```python
from build123d import *

# Parameters (mm, degrees)
F2_R     = 2
F3_DEPTH = 1.5875


with BuildPart() as f3:
    # F2 (on offset) → F3 (new body)
    with BuildSketch(Plane.XZ.offset(22.225)):
        with BuildLine():
            Line((-64.792564, 23.8125), (-111.76, 23.8125))
            ThreePointArc((-111.76, 23.8125), (-130.205083, 15.060347), (-135.09139, -4.7625))
            Line((-135.09139, -4.7625), (-93.367564, -4.7625))
            Line((-93.367564, -4.7625), (-64.792564, 23.8125))
        make_face()
        with Locations((-111.76, 0)):
            Circle(F2_R, mode=Mode.SUBTRACT)
    extrude(amount=-F3_DEPTH)


solid = f3.part
```
Geometry check sheet. Reference: the model listing, model coordinates, mm. Give positions to 0.01 mm unless a question says otherwise; leave off trailing zeros. Order: outer loops, then holes, each group sorted by start corner. A loop starts at its lowest first (then second) coordinate and runs counter-clockwise, first axis right, second up. Notation, with made-up numbers: (-35.5, -1.75) - (17.5, -1.75) arc R20 cw to (17.5, 32.25) - close; hole circle Ø6 at (-14.75, -4.5). An arc over 180 degrees is marked (long way). Write item = value, one per line. Start each with the question number.
1) Draft check along X on faces 1 (the flat face through (-79.28, -21.442, 9.325)), 2 (the cylindrical face through (-109.852, -21.442, 0.601)), 3 (the flat face through (-88, -21, 23.812)), 4 (the cylindrical face through (-130.017, -21.442, 15.288)). Enter one of: released by +X, released by -X, zero draft, split by the parting line, or undercut.
2) Section check D-D (z = 8.75). Enter the section's corners in (x, y) (1 decimal), then the cut area to 3 significant figures.
3) Gauge pin test, flat ends, axial feed: pin 1 Ø4 at (x, z) = (-83.5, 0) entering from -Y; pin 2 Ø5 at (x, z) = (-111.76, 0) entering from +Y. Record the tip position at first contact, or that the pin passes through.
4) Section check C-C (x = -110.5). Enter the section's corners in (y, z) (1 decimal).
5) Section check B-B (y = -21.3). Enter the section's corners in (x, z) (1 decimal), then the cut area to 3 significant figures.
6) Section check A-A (z = 0). Enter the section's corners in (x, y) (1 decimal), then the cut area to 3 significant figures.
7) Scan lines: L1, parallel to Z at x = -111.76, y = -21.75; L2, parallel to X at y = -21.7, z = -1.5; L3, parallel to Z at x = -113, y = -21.2. Record each from-to range of solid material in increasing order.
Geometry check:
q1.face_1 = released by +X
q1.face_2 = undercut
q1.face_3 = zero draft
q1.face_4 = released by -X
q2.outline = (-133.9, -22.2) - (-79.9, -22.2) - (-79.9, -20.6) - (-133.9, -20.6) - close
q2.area = 85.8 mm2
q3.pin_1 = through
q3.pin_2 = -20.64
q4.outline = (-22.2, -4.8) - (-20.6, -4.8) - (-20.6, -1.6) - (-22.2, -1.6) - close; (-22.2, 1.6) - (-20.6, 1.6) - (-20.6, 23.8) - (-22.2, 23.8) - close
q5.outline = (-135.1, -4.8) - (-93.4, -4.8) - (-64.8, 23.8) - (-111.8, 23.8) arc R23.8 ccw to start; hole circle Ø4 at (-111.8, 0)
q5.area = 1,480 mm2
q6.outline = (-135.6, -22.2) - (-113.8, -22.2) - (-113.8, -20.6) - (-135.6, -20.6) - close; (-109.8, -22.2) - (-88.6, -22.2) - (-88.6, -20.6) - (-109.8, -20.6) - close
q6.area = 68.2 mm2
q7.L1 = -4.76 to -2, 2 to 23.81
q7.L2 = -135.53 to -113.08, -110.44 to -90.11
q7.L3 = -4.76 to -1.57, 1.57 to 23.78
